Geometry check sheet. Reference: drawing and pictorial views, mm from the part's lowest x, y, z. Give positions to 0.01 mm unless a question says otherwise; leave off trailing zeros. Write each loop counter-clockwise with the first axis right and the second up, starting at its lowest first coordinate (ties: lowest second). Pieces come first, ordered by that corner, then holes. Notation, with made-up numbers: M 83,50 L 92,50 A20 cw 92,88 Z; hole C -1.75,-38 d6. An arc over 180 degrees is marked long. One line per item, written item: value. Start each with the question number.
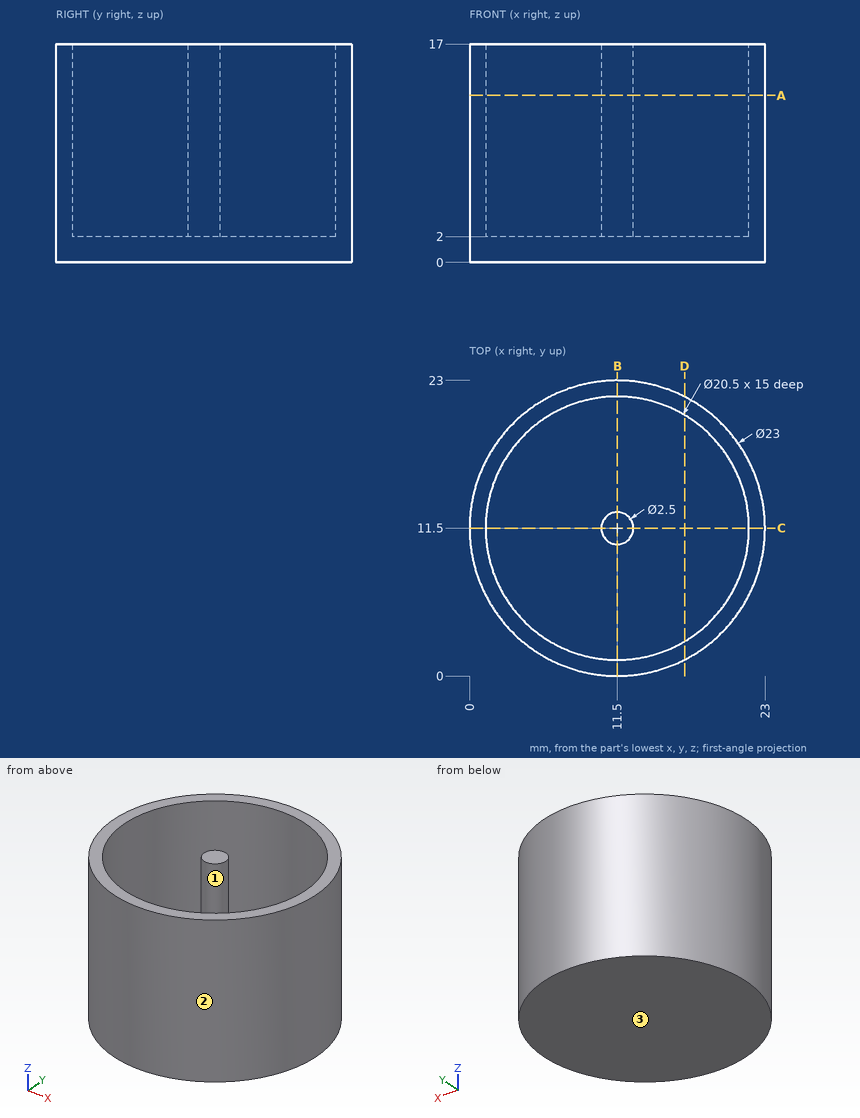
1) Draft check along X on the marked faces 1, 2 and 3. Enter one of: released by +X, released by -X, zero draft, split by the parting line, or undercut.
2) Cross-section at A-A (z = 13). Record the boundary of the cut face in (x, y), plus the area to 3 significant figures.
3) Gauge pin test, flat ends, axial feed: pin 1 (8 mm diameter, centred on x = 19.5, z = 9.5, fed in from -Y); pin 2 (6 mm diameter, centred on x = 17.5, z = 12, fed in from -Y); pin 3 (1.5 mm diameter, centred on x = 14, z = 13.5, fed in from -Y). Record the tip position at first contact, or that the pin passes through.
4) Cross-section at B-B (x = 11.5). Record the boundary of the cut face in (y, z), plus the area to 3 significant figures.
5) Material ranges on L1, parallel to Y at x = 11.5, z = 8.75; L2, parallel to X at y = 15, z = 9; L3, parallel to Y at x = 15.75, z = 10.5, recorded low to high. Write a range as from..to.
6) Cross-section at D-D (x = 16.75). Record the boundary of the cut face in (y, z).
Data:
1. face 1: undercut
1. face 2: split by the parting line
1. face 3: zero draft
2. outline: C 11.5,11.5 d23; C 11.5,11.5 d2.5; hole C 11.5,11.5 d20.5
2. area: 90.3 mm2
3. pin 1: stops at y = 0.72
3. pin 2: stops at y = 0.4
3. pin 3: stops at y = 0.13
4. outline: M 0,0 L 23,0 L 23,17 L 21.75,17 L 21.75,2 L 12.75,2 L 12.75,17 L 10.25,17 L 10.25,2 L 1.25,2 L 1.25,17 L 0,17 Z
4. area: 121 mm2
5. L1: y = 0..1.25, 10.25..12.75, 21.75..23
5. L2: x = 0.55..1.87, 21.13..22.45
5. L3: y = 0.81..2.17, 20.83..22.19
6. outline: M 1.27,0 L 21.73,0 L 21.73,17 L 20.3,17 L 20.3,2 L 2.7,2 L 2.7,17 L 1.27,17 Z
